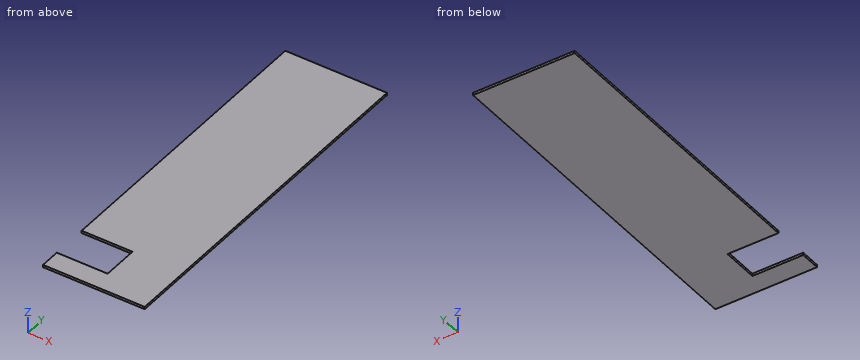
Autodesk Inventor part; units mm, degrees
ref_plane "YZ Plane" through (0, 0, 0) normal (1, 0, 0) x (0, 1, 0)
ref_plane "XZ Plane" through (0, 0, 0) normal (0, 1, 0) x (-1, 0, 0)
ref_plane "XY Plane" through (0, 0, 0) normal (0, 0, 1) x (1, 0, 0)
sketch "Sketch2" plane through (0, 0, 0) normal (0, 0, 1) x (1, 0, 0)
  line L0 (0, 0) -> (126, 0)
  line L1 (126, 0) -> (126, 439)
  line L2 (126, 439) -> (0, 439)
  line L3 (0, 439) -> (0, 0)
  line L4 (0, 25) -> (63, 25)
  line L5 (63, 0) -> (0, 0)
  line L6 (0, 0) -> (0, 25)
  line L7 (63, 25) -> (63, 70)
  line L8 (63, 70) -> (0, 70)
  point P0 (63, 47.5)
  dimension "d0" = 126
  dimension "d1" = 439
  dimension "d2" = 25
  dimension "d3" = 45
  dimension "d4" = 63
extrude "Extrusion1" add sketch "Sketch2" along normal blind 3 contours L3 L4 L7 L8 L2 L1 L0
properties part number "ackleryk" material "PMMA Plastic"
Design review of the part built by this model. Coordinates are the model's own, in mm. Round coordinates to 2 decimals unless told otherwise and drop trailing zeros. Write each loop counter-clockwise with the first axis right and the second up, starting at its lowest first coordinate (ties: lowest second). Pieces come first, ordered by that corner, then holes. Notation, with made-up numbers: (60, 79) - (105, 79) arc R21 ccw to (105, 86) - close; hole circle Ø5 at (63, 75). An arc over 180 degrees is marked (long way). Return JSON: item names as keys, results as strings. Group by question number.
Item 1: We need section B-B on x = 17.5. Write out the cut boundary in (y, z).
Item 2: Insertion check: P1, Ø0.9, axis at y = 39.5, z = 1, coming from the -X side; P2, Ø1.5, axis at x = 53.5, z = 0.5, coming from the -Y side. Each pin has a flat end and moves straight along its axis. Give the tip position at first contact, or say it passes through.
Item 3: We need section C-C on y = 48. Write out the cut boundary in (x, z).
Item 4: We need section A-A on z = 1.4. Write out the cut boundary in (x, y).
Item 5: For probe 1 along Y at (x, z) = (62, 2.4); probe 2 along X at (y, z) = (64, 0.95), list the stretches that pass through material, from the lowest coordinate up. Write a range as [from, to].
Model answer:
{
 "1": {"outline": "(0, 0) - (25, 0) - (25, 3) - (0, 3) - close; (70, 0) - (439, 0) - (439, 3) - (70, 3) - close"},
 "2": {"P1": "stops at x = 63", "P2": "stops at y = 0"},
 "3": {"outline": "(63, 0) - (126, 0) - (126, 3) - (63, 3) - close"},
 "4": {"outline": "(0, 0) - (126, 0) - (126, 439) - (0, 439) - (0, 70) - (63, 70) - (63, 25) - (0, 25) - close"},
 "5": {"probe 1": "y = [0, 25], [70, 439]", "probe 2": "x = [63, 126]"}
}
